from build123d import *

# Parameters (mm, degrees)
SKETCH1_W                 = 100
SKETCH1_H                 = 100
BOSS_EXTRUDE1_DEPTH       = 60
SKETCH2_W                 = 98
SKETCH2_H                 = 98
CUT_EXTRUDE1_DEPTH        = 60
SKETCH3_R                 = 1
CUT_EXTRUDE2_DEPTH        = 125
CUT_EXTRUDE3_DEPTH        = 10
BOSS_EXTRUDE4_START       = 50
BOSS_EXTRUDE4_OUTLINE_W   = 39.858082606
BOSS_EXTRUDE4_OUTLINE_H   = 40
BOSS_EXTRUDE4_OUTLINE_W_2 = 38.374033315
BOSS_EXTRUDE4_OUTLINE_H_2 = 38.356376399
BOSS_EXTRUDE4_OUTLINE_W_3 = 1.151682465
BOSS_EXTRUDE4_OUTLINE_H_3 = 6.68708673
BOSS_EXTRUDE4_OUTLINE_W_4 = 1.169732075
BOSS_EXTRUDE4_OUTLINE_R   = 1.29952059
BOSS_EXTRUDE4_OUTLINE_W_5 = 3.781559684
BOSS_EXTRUDE4_OUTLINE_H_4 = 1.155970525
BOSS_EXTRUDE4_OUTLINE_W_6 = 3.781559683
BOSS_EXTRUDE4_DEPTH       = 2
SKETCH9_R                 = 3.5
CUT_EXTRUDE4_DEPTH        = 10
FILLET1_R                 = 1


# Read off the part's stored shape, not the designer's step: Boss-Extrude4
with BuildPart() as part:
    # Sketch1 → Boss-Extrude1 (new body)
    with BuildSketch(Plane(origin=(0, 0, 0), x_dir=(1, 0, 0), z_dir=(0, 1, 0))):
        Rectangle(SKETCH1_W, SKETCH1_H)
    extrude(amount=BOSS_EXTRUDE1_DEPTH)

    # Sketch2 → Cut-Extrude1 (cut)
    with BuildSketch(Plane(origin=(0, 60, 0), x_dir=(1, 0, 0), z_dir=(0, 1, 0))):
        Rectangle(SKETCH2_W, SKETCH2_H)
    extrude(amount=-CUT_EXTRUDE1_DEPTH, mode=Mode.SUBTRACT)

    # Sketch3 → Cut-Extrude2 (cut)
    with BuildSketch(Plane(origin=(50, 0, 0), x_dir=(0, 0, -1), z_dir=(1, 0, 0))):
        with BuildLine():
            ThreePointArc((-24, 57.5), (-25, 58.5), (-26, 57.5))
            Line((-26, 57.5), (-24, 57.5))
        make_face()
        with BuildLine():
            Line((-24, 57.5), (-26, 57.5))
            ThreePointArc((-26, 57.5), (-25, 56.5), (-24, 57.5))
        make_face()
        with Locations((25, 57.5)):
            Circle(SKETCH3_R)
        with Locations((-25, 2.5)):
            Circle(SKETCH3_R)
        with Locations((25, 2.5)):
            Circle(SKETCH3_R)
    extrude(amount=-CUT_EXTRUDE2_DEPTH, mode=Mode.SUBTRACT)

    # Sketch5 → Cut-Extrude3 (cut)
    with BuildSketch(Plane.ZY.offset(50)):
        with BuildLine():
            ThreePointArc((3.25, 17.5), (2.298097039, 19.798097039), (0, 20.75))
            Line((0, 20.75), (0, 14.25))
            ThreePointArc((0, 14.25), (2.298097039, 15.201902961), (3.25, 17.5))
        make_face()
        with BuildLine():
            Line((0, 14.25), (0, 20.75))
            ThreePointArc((0, 20.75), (-3.25, 17.5), (0, 14.25))
        make_face()
    extrude(amount=-CUT_EXTRUDE3_DEPTH, mode=Mode.SUBTRACT)

    # Boss-Extrude4 outline → Boss-Extrude4 (add)
    # profile 1 of 13: a face of its own
    with BuildSketch(Plane.XY.offset(BOSS_EXTRUDE4_START)):
        with Locations((0, 25)):
            Rectangle(BOSS_EXTRUDE4_OUTLINE_W, BOSS_EXTRUDE4_OUTLINE_H)
        with Locations((-0.051593215, 24.997020999)):
            Rectangle(BOSS_EXTRUDE4_OUTLINE_W_2, BOSS_EXTRUDE4_OUTLINE_H_2, mode=Mode.SUBTRACT)
    # profile 2 of 13: a face of its own
    with BuildSketch(Plane.XY.offset(BOSS_EXTRUDE4_START)):
        with BuildLine():
            Line((-9.922016309, 32.280172221), (-9.922016309, 33.453564236))
            Line((-9.922016309, 33.453564236), (-13.93029333, 33.453564236))
            ThreePointArc((-13.93029333, 33.453564236), (-14.849532145, 33.072803052), (-15.23029333, 32.153564236))
            Line((-15.23029333, 32.153564236), (-15.23029333, 28.064542243))
            ThreePointArc((-15.23029333, 28.064542243), (-14.849532146, 27.145303428), (-13.93029333, 26.764542243))
            Line((-13.93029333, 26.764542243), (-9.925370196, 26.764542243))
            Line((-9.925370196, 26.764542243), (-9.925370196, 27.933655334))
            Line((-9.925370196, 27.933655334), (-13.55690574, 27.933655334))
            ThreePointArc((-13.55690574, 27.933655334), (-13.910459131, 28.080101943), (-14.05690574, 28.433655334))
            Line((-14.05690574, 28.433655334), (-14.05690574, 31.880172221))
            ThreePointArc((-14.05690574, 31.880172221), (-13.939748452, 32.163014933), (-13.65690574, 32.280172221))
            Line((-13.65690574, 32.280172221), (-9.922016309, 32.280172221))
        make_face()
    # profile 3 of 13: a face of its own
    with BuildSketch(Plane.XY.offset(BOSS_EXTRUDE4_START)):
        with Locations((-6.175417948, 30.110020871)):
            Rectangle(BOSS_EXTRUDE4_OUTLINE_W_3, BOSS_EXTRUDE4_OUTLINE_H_3)
    # profile 4 of 13: a face of its own
    with BuildSketch(Plane.XY.offset(BOSS_EXTRUDE4_START)):
        Polygon((-1.00100917, 26.766477506), (-1.00100917, 33.453564236), (-2.170113717, 33.453564236), (-2.170113717, 30.935634342), (-5.349717596, 30.935634342), (-5.349717596, 29.768397912), (-2.170113717, 29.768397912), (-2.170113717, 26.766477506), align=None)
    # profile 5 of 13: a face of its own
    with BuildSketch(Plane.XY.offset(BOSS_EXTRUDE4_START)):
        with Locations((4.358014237, 30.110020871)):
            Rectangle(BOSS_EXTRUDE4_OUTLINE_W_4, BOSS_EXTRUDE4_OUTLINE_H_3)
    # profile 6 of 13: a face of its own
    with BuildSketch(Plane.XY.offset(BOSS_EXTRUDE4_START)):
        with BuildLine():
            Line((9.038474855, 26.766477506), (9.954821181, 26.766477506))
            Line((9.954821181, 26.766477506), (9.954821181, 31.435250737))
            ThreePointArc((9.954821181, 31.435250737), (10.237464032, 31.982611448), (10.746519943, 32.329530473))
            ThreePointArc((10.746519943, 32.329530473), (15.159384473, 32.918290446), (10.721414833, 33.271046936))
            ThreePointArc((10.721414833, 33.271046936), (9.619160753, 32.646851071), (9.038474855, 31.521067599))
            Line((9.038474855, 31.521067599), (9.038474855, 26.766477506))
        make_face()
        with Locations((12.921637239, 32.858621929)):
            Circle(BOSS_EXTRUDE4_OUTLINE_R, mode=Mode.SUBTRACT)
    # profile 7 of 13: a face of its own
    with BuildSketch(Plane.XY.offset(BOSS_EXTRUDE4_START)):
        Polygon((15.358270934, 20.30132248), (15.358270934, 21.474568974), (10.074546624, 21.474568974), (10.074546624, 14.78091915), (15.358270934, 14.78091915), (15.358270934, 15.94490899), (11.24592521, 15.94490899), (11.24592521, 20.30132248), align=None)
    # profile 8 of 13: a face of its own
    with BuildSketch(Plane.XY.offset(BOSS_EXTRUDE4_START)):
        Polygon((7.108297958, 21.474568974), (1.824573649, 21.474568974), (1.824573649, 14.78091915), (7.108297958, 14.78091915), (7.108297958, 15.94490899), (2.995952235, 15.94490899), (2.995952235, 20.30132248), (7.108297958, 20.30132248), align=None)
    # profile 9 of 13: a face of its own
    with BuildSketch(Plane.XY.offset(BOSS_EXTRUDE4_START)):
        with Locations((13.387987428, 18.375193575)):
            Rectangle(BOSS_EXTRUDE4_OUTLINE_W_5, BOSS_EXTRUDE4_OUTLINE_H_4)
    # profile 10 of 13: a face of its own
    with BuildSketch(Plane.XY.offset(BOSS_EXTRUDE4_START)):
        with Locations((5.138014453, 18.375193575)):
            Rectangle(BOSS_EXTRUDE4_OUTLINE_W_6, BOSS_EXTRUDE4_OUTLINE_H_4)
    # profile 11 of 13: a face of its own
    with BuildSketch(Plane.XY.offset(BOSS_EXTRUDE4_START)):
        with BuildLine():
            Line((-6.283421644, 14.927747144), (-6.283421644, 19.478331399))
            ThreePointArc((-6.283421644, 19.478331399), (-6.000778792, 20.025692111), (-5.491722882, 20.372611136))
            ThreePointArc((-5.491722882, 20.372611136), (-1.078858352, 20.961371104), (-5.516827991, 21.314127598))
            ThreePointArc((-5.516827991, 21.314127598), (-6.619082072, 20.689931733), (-7.19976797, 19.564148262))
            Line((-7.19976797, 19.564148262), (-7.19976797, 14.927747144))
            Line((-7.19976797, 14.927747144), (-6.283421644, 14.927747144))
        make_face()
        with Locations((-3.316605586, 20.901702592)):
            Circle(BOSS_EXTRUDE4_OUTLINE_R, mode=Mode.SUBTRACT)
    # profile 12 of 13: a face of its own
    with BuildSketch(Plane.XY.offset(BOSS_EXTRUDE4_START)):
        Polygon((-3.743380156, 18.2010008), (-4.392168827, 17.55221213), (-1.75326942, 14.913312723), (-1.104480749, 15.562101393), align=None)
    # profile 13 of 13: a face of its own
    with BuildSketch(Plane.XY.offset(BOSS_EXTRUDE4_START)):
        Polygon((-15.305624402, 21.469309136), (-15.305624402, 20.296062642), (-13.00828814, 20.296062642), (-13.00828814, 14.784735536), (-11.838556065, 14.784735536), (-11.838556065, 20.296062642), (-9.582967691, 20.296062642), (-9.582967691, 21.469309136), align=None)
    extrude(amount=BOSS_EXTRUDE4_DEPTH)

    # Sketch9 → Cut-Extrude4 (cut)
    with BuildSketch(Plane.XY.offset(50)):
        with Locations((-40, 46)):
            Circle(SKETCH9_R)
    extrude(amount=-CUT_EXTRUDE4_DEPTH, mode=Mode.SUBTRACT)

    # Fillet1
    fillet1_edges = [part.edges().sort_by_distance(p)[0] for p in [
        (50, 30, 50),
        (-50, 30, 50),
        (-50, 30, -50),
        (50, 30, -50),
    ]]
    fillet(fillet1_edges, radius=FILLET1_R)


solid = part.part
Can you work these out from the model? Positions are in its coordinate system, mm. A direction names the side the tool comes from. Coordinates: 2 decimals unless noted, no trailing zeros. Loops run counter-clockwise (first coordinate to the right, second up) from the corner with the lowest first, then second, coordinate; pieces in that order, holes last. Notation, with made-up numbers: (66, 16) - (115, 16) arc R19 ccw to (115, 39) - close; hole circle Ø2 at (0, 63.25). An arc over 180 degrees is marked (long way). Put each result on its own line as item: value. Start each with the question number.
Item 1: If I drill on line 1 along Y through (x, z) = (49.45, 25); line 2 along Z through (x, y) = (10, 57), over which ranges is the centre line in solid material (lowest first)?
Item 2: Suppose I cut it at A-A (x = -40). Please give me the cut outline in (y, z).
Item 3: If we mould it in two halves opening along X, with no side actions, what happens to faces 1 (the face through (15.16, 32.83, 50.99)), 2 (the face through (2.7, 18.2, 52)), 3 (the face through (-42.58, 48.365, 49.507)), 4 (the face through (-50, 30, 1))? For each: +X half, -X half, draft (parallel to the pull), parting line (faces both ways), or undercut.
Item 4: For pin 1 (1.6 mm diameter, centred on x = 3.5, z = 51, fed in from +Y); pin 2 (1.8 mm diameter, centred on y = 2.5, z = 25, fed in from +X); pin 3 (1 mm diameter, centred on x = -14, z = 51.5, fed in from -Y); pin 4 (0.6 mm diameter, centred on y = 31.5, z = 51.5, fed in from +X), each with a flat end and sliding along its axis, tell me the tip position at first contact or that it passes through.
Item 5: Suppose I cut it at D-D (y = 39). Please give me the cut outline in (x, z).
Item 6: Which directions (+Z, -Z, +X, -X, +Y, -Y) give clear straight access to the entire face, cutting with the end or side of a thin tool? Please do faces 5 (the face through (-3, 21, 50)), 6 (the face through (11.4, 31.9, 52)).
Item 7: Suppose I cut it at C-C (x = 40). Please give me the cut outline in (y, z).
Item 8: Suppose I cut it at B-B (z = 11). Please give me the cut outline in (x, y), and give its area (3 significant figures).
Here are the results:
1. line 1: 0 to 1.5, 3.5 to 56.5, 58.5 to 60
1. line 2: -50 to -49, 49 to 50
2. outline: (0, -50) - (60, -50) - (60, -49) - (0, -49) - close; (0, 49) - (42.5, 49) - (42.5, 50) - (0, 50) - close; (49.5, 49) - (60, 49) - (60, 50) - (49.5, 50) - close
3. face 1: undercut
3. face 2: draft
3. face 3: undercut
3. face 4: -X half
4. pin 1: y = 45
4. pin 2: through
4. pin 3: y = 5
4. pin 4: x = 19.93
5. outline: (-50, -49) arc R1 ccw to (-49, -50) - (49, -50) arc R1 ccw to (50, -49) - (50, 49) arc R1 ccw to (49, 50) - (19.93, 50) - (19.93, 52) - (19.14, 52) - (19.14, 50) - (-19.24, 50) - (-19.24, 52) - (-19.93, 52) - (-19.93, 50) - (-49, 50) arc R1 ccw to (-50, 49) - close; hole (-49, -49) - (49, -49) - (49, 49) - (-49, 49) - close
6. face 5: +Z
6. face 6: +Z, +X, -X, +Y, -Y
7. outline: (0, -50) - (60, -50) - (60, -49) - (0, -49) - close; (0, 49) - (60, 49) - (60, 50) - (0, 50) - close
8. outline: (-50, 0) - (-49, 0) - (-49, 60) - (-50, 60) - close; (49, 0) - (50, 0) - (50, 60) - (49, 60) - close
8. area: 120 mm²
